For this review, take the finished solid that the model builds, in its own axes (mm). A direction names the side the tool comes from. Coordinates: 2 decimals unless noted, no trailing zeros. Loops run counter-clockwise (first coordinate to the right, second up) from the corner with the lowest first, then second, coordinate; pieces in that order, holes last. Notation, with made-up numbers: (11, 17) - (25, 17) arc R9 cw to (25, 27) - close; hole circle Ø3 at (-7, 68). An arc over 180 degrees is marked (long way). Answer as a JSON object with one key per item and string values. Group by question number.
Item 1: To check wall thickness, follow line 1 (Y direction, x = 349, z = 24.5) (3 decimals); line 2 (X direction, y = 2.5, z = 26). State the ranges of each line that lie inside material, in increasing order.
Item 2: We need section B-B (z = 17). Give the boundary of the cut face in (x, y) (3 decimals), then the cut area to 3 significant figures.
Item 3: Clearance check with flat-ended pins moving along their axes: pin 1 (8.5 mm diameter, centred on x = 285.5, y = 12.5, fed in from +Z) (3 decimals); pin 2 (4 mm diameter, centred on x = 186, z = 5.5, fed in from +Y) (3 decimals); pin 3 (6 mm diameter, centred on y = 16, z = 5.5, fed in from -X). State where each tip first meets the part, or that it passes through.
Item 4: We need section A-A (x = 349.5). Give the boundary of the cut face in (y, z) (3 decimals), then the cut area to 3 significant figures.
Item 5: Tool access review of faces 1 (the flat face through (251, 0, 16)), 2 (the flat face through (251, 3.175, 18)): name each direction out of +Z, -Z, +X, -X, +Y, -Y from which nothing blocks a thin tool from reaching the whole face with its end or side.
from build123d import *

# Parameters (mm, degrees)
BOSS_EXTRUDE1_DEPTH          = 510
CHAMFER6_SIZE                = 31.75
CHAMFER7_SIZE                = 31.75
TOPHOLES_SKETCH3_R           = 1.5875
TOPHOLES_CUT_EXTRUDE2_DEPTH  = 512.785690622
SIDEHOLES_SKETCH4_R          = 1.5875
SIDEHOLES_SKETCH4_R_2        = 2
SIDEHOLES_CUT_EXTRUDE3_DEPTH = 512.785690622


with BuildPart() as part:
    # Sketch1 → Boss-Extrude1 (new body)
    with BuildSketch(Plane(origin=(0, 0, 0), x_dir=(0, 0, -1), z_dir=(1, 0, 0))):
        Polygon((0, 0), (-31.75, 0), (-31.75, 3.175), (-3.175, 3.175), (-3.175, 31.75), (0, 31.75), align=None)
    extrude(amount=BOSS_EXTRUDE1_DEPTH)

    # Chamfer6
    chamfer6_edges = [part.edges().sort_by_distance(p)[0] for p in [
        (510, 1.5875, 31.75),
    ]]
    chamfer(chamfer6_edges, length=CHAMFER6_SIZE - 0.0001)  # a hair under: the kernel refuses the full size

    # Chamfer7
    chamfer7_edges = [part.edges().sort_by_distance(p)[0] for p in [
        (0, 1.5875, 31.75),
    ]]
    chamfer(chamfer7_edges, length=CHAMFER7_SIZE - 0.0001)  # a hair under: the kernel refuses the full size

    # TopHoles-Sketch3 → TopHoles-Cut-Extrude2 (cut, through all)
    with BuildSketch(Plane(origin=(0, 3.175, 0), x_dir=(1, 0, 0), z_dir=(0, 1, 0))):
        with Locations(Location((58.7375, -23.8125, 0), (0, 0, 270))):
            Circle(TOPHOLES_SKETCH3_R)
        with Locations(Location((451.2625, -23.8125, 0), (0, 0, 270))):
            Circle(TOPHOLES_SKETCH3_R)
        with Locations(Location((451.2625, -11.1125, 0), (0, 0, 270))):
            Circle(TOPHOLES_SKETCH3_R)
        with Locations(Location((58.7375, -11.1125, 0), (0, 0, 270))):
            Circle(TOPHOLES_SKETCH3_R)
        with Locations(Location((486.1875, -11.1125, 0), (0, 0, 270))):
            Circle(TOPHOLES_SKETCH3_R)
        with Locations(Location((23.8125, -11.1125, 0), (0, 0, 270))):
            Circle(TOPHOLES_SKETCH3_R)
        with Locations(Location((127.5, -11.1125, 0), (0, 0, 270))):
            Circle(TOPHOLES_SKETCH3_R)
        with Locations(Location((255, -11.1125, 0), (0, 0, 270))):
            Circle(TOPHOLES_SKETCH3_R)
        with Locations(Location((382.5, -11.1125, 0), (0, 0, 270))):
            Circle(TOPHOLES_SKETCH3_R)
    extrude(amount=-TOPHOLES_CUT_EXTRUDE2_DEPTH, mode=Mode.SUBTRACT)

    # SideHoles-Sketch4 → SideHoles-Cut-Extrude3 (cut, through all)
    with BuildSketch(Plane.XY.offset(3.175)):
        with Locations((11.1125, 23.8125)):
            Circle(SIDEHOLES_SKETCH4_R)
        with Locations((489.3625, 23.8125)):
            Circle(SIDEHOLES_SKETCH4_R)
        with Locations((20.6375, 23.8125)):
            Circle(SIDEHOLES_SKETCH4_R)
        with Locations((498.8875, 23.8125)):
            Circle(SIDEHOLES_SKETCH4_R)
        with Locations((11.1125, 11.1125)):
            Circle(SIDEHOLES_SKETCH4_R)
        with Locations((20.6375, 11.1125)):
            Circle(SIDEHOLES_SKETCH4_R)
        with Locations((489.3625, 11.1125)):
            Circle(SIDEHOLES_SKETCH4_R)
        with Locations((498.8875, 11.1125)):
            Circle(SIDEHOLES_SKETCH4_R)
        with Locations((200, 11.1125)):
            Circle(SIDEHOLES_SKETCH4_R_2)
        with Locations((215, 11.1125)):
            Circle(SIDEHOLES_SKETCH4_R_2)
        with Locations((230, 11.1125)):
            Circle(SIDEHOLES_SKETCH4_R_2)
        with Locations((127.5, 11.1125)):
            Circle(SIDEHOLES_SKETCH4_R)
        with Locations((382.5, 11.1125)):
            Circle(SIDEHOLES_SKETCH4_R)
    extrude(amount=-SIDEHOLES_CUT_EXTRUDE3_DEPTH, mode=Mode.SUBTRACT)


solid = part.part
Check sheet entries:
{
 "1": {"line 1": "y = 0 to 3.175", "line 2": "x = 26 to 484"},
 "2": {"outline": "(17, 0) - (493, 0) - (493, 3.175) - (17, 3.175) - close", "area": "1,510 mm2"},
 "3": {"pin 1": "stops at z = 3.175", "pin 2": "stops at y = 3.175", "pin 3": "stops at x = 2.5"},
 "4": {"outline": "(0, 0) - (31.75, 0) - (31.75, 3.175) - (3.175, 3.175) - (3.175, 31.75) - (0, 31.75) - close", "area": "192 mm2"},
 "5": {"face 1": "+Z, -Z, +X, -X, -Y", "face 2": "+Z, +X, -X, +Y"}
}
